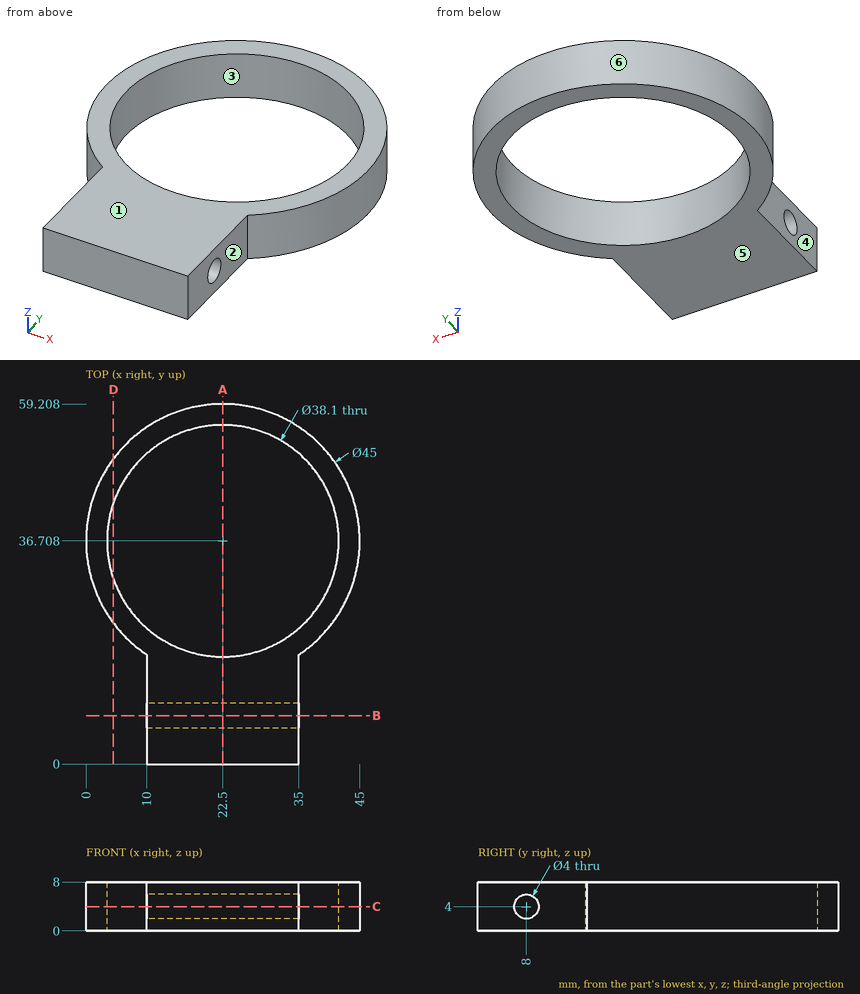
Source: three-view drawing plus pictorial views. Frame: mm from the lowest corner of the part. A direction names the side the tool comes from. Give positions to 0.01 mm unless a question says otherwise; leave off trailing zeros. Order: outer loops, then holes, each group sorted by start corner. A loop starts at its lowest first (then second) coordinate and runs counter-clockwise, first axis right, second up. Notation, with made-up numbers: (28.5, 30.25) - (56.5, 30.25) arc R19 ccw to (56.5, 51.25) - close; hole circle Ø11 at (-36.75, -1). An arc over 180 degrees is marked (long way). Answer as a JSON object with one key per item and string values. Group by question number.
Q1. Cut plane A-A, the plane x = 22.5. Output: boundary loops of the cut face in (y, z).
Q2. Line query: probe 1 along Y at (x, z) = (22.5, 4.25) (1 decimal); probe 2 along Z at (x, y) = (18.5, 8); probe 3 along Y at (x, z) = (22.5, 4.5). Output: solid intervals per line, ascending.
Q3. Cut plane B-B, the plane y = 8. Output: boundary loops of the cut face in (x, z).
Q4. Cut plane C-C, the plane z = 4. Output: boundary loops of the cut face in (x, y).
Q5. Set-up query: the marked faces 1 and 2. Return all of +Z, -Z, +X, -X, +Y, -Y with unobstructed straight access to the full face (end or side cutting, diameter ignored); none if empty.
Q6. Mould query, pull axis X, two halves, no side actions, for the marked faces 3, 4, 5 and 6. Classes: pulls with the +X half, pulls with the -X half, needs draft (parallel to the pull), parting line crosses it, or undercut.
Q7. First-contact query: pin 1 Ø3 at (x, z) = (38, 2) entering from -Y (1 decimal); pin 2 Ø1 at (y, z) = (6.5, 5.5) entering from -X; pin 3 Ø4 at (y, z) = (6, 5) entering from +X. Flat tips, straight axial feed; report the tip coordinate or a pass-through.
Q8. Cut plane D-D, the plane x = 4.5. Output: boundary loops of the cut face in (y, z) (1 decimal).
Results:
{
 "1": {"outline": "(0, 0) - (17.66, 0) - (17.66, 8) - (0, 8) - close; (55.76, 0) - (59.21, 0) - (59.21, 8) - (55.76, 8) - close; hole circle Ø4 at (8, 4)"},
 "2": {"probe 1": "0 to 6, 10 to 17.7, 55.8 to 59.2", "probe 2": "0 to 2, 6 to 8", "probe 3": "0 to 6.06, 9.94 to 17.66, 55.76 to 59.21"},
 "3": {"outline": "(10, 0) - (35, 0) - (35, 2) - (10, 2) - close; (10, 6) - (35, 6) - (35, 8) - (10, 8) - close"},
 "4": {"outline": "(10, 0) - (35, 0) - (35, 6) - (10, 6) - close; (10, 10) - (35, 10) - (35, 18) arc R22.5 ccw (long way) to (10, 18) - close; hole circle Ø38.1 at (22.5, 36.71)"},
 "5": {"face 1": "+Z, +X, -X, +Y, -Y", "face 2": "+Z, -Z, +X, -Y"},
 "6": {"face 3": "undercut", "face 4": "pulls with the -X half", "face 5": "needs draft", "face 6": "parting line crosses it"},
 "7": {"pin 1": "y = 19.1", "pin 2": "x = 10", "pin 3": "x = 35"},
 "8": {"outline": "(23.2, 0) - (30.5, 0) - (30.5, 8) - (23.2, 8) - close; (42.9, 0) - (50.2, 0) - (50.2, 8) - (42.9, 8) - close"}
}
